Read the model definition and answer for the solid it produces. Units are mm, in the model's axes. Coordinates: 2 decimals unless noted, no trailing zeros.
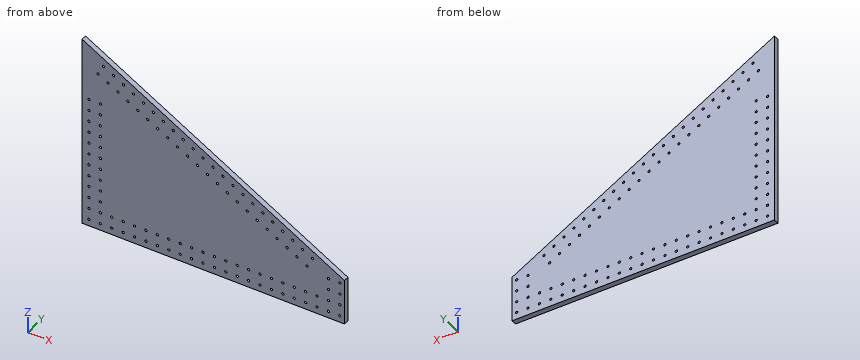
from build123d import *

# Parameters (mm, degrees)
F1_DEPTH = 12
F2_R     = 2.5527
F3_DEPTH = 508


with BuildPart() as f1:
    # F0 (on Front) → F1 (new body)
    with BuildSketch(Plane.XZ):
        Polygon((511.232538, -258.696949), (-72.967462, 69.018931), (-72.967462, -360.296949), (511.232538, -360.296949), align=None)
    extrude(amount=F1_DEPTH)

    # F2 (on face) → F3 (cut)
    with BuildSketch(Plane.XZ.offset(12)):
        with Locations((-57.714762, -345.044249)):
            Circle(F2_R)
        with Locations((-57.714762, -319.644249)):
            Circle(F2_R)
        with Locations((-57.714762, -294.244249)):
            Circle(F2_R)
        with Locations((-57.714762, -268.844249)):
            Circle(F2_R)
        with Locations((-57.714762, -243.444249)):
            Circle(F2_R)
        with Locations((-57.714762, -218.044249)):
            Circle(F2_R)
        with Locations((-57.714762, -192.644249)):
            Circle(F2_R)
        with Locations((-57.714762, -167.244249)):
            Circle(F2_R)
        with Locations((-57.714762, -141.844249)):
            Circle(F2_R)
        with Locations((-57.714762, -116.444249)):
            Circle(F2_R)
        with Locations((-57.714762, -91.044249)):
            Circle(F2_R)
        with Locations((-57.714762, -65.644249)):
            Circle(F2_R)
        with Locations((-32.314762, -345.044249)):
            Circle(F2_R)
        with Locations((-32.314762, -319.644249)):
            Circle(F2_R)
        with Locations((-32.314762, -294.244249)):
            Circle(F2_R)
        with Locations((-32.314762, -268.844249)):
            Circle(F2_R)
        with Locations((-32.314762, -243.444249)):
            Circle(F2_R)
        with Locations((-32.314762, -218.044249)):
            Circle(F2_R)
        with Locations((-32.314762, -192.644249)):
            Circle(F2_R)
        with Locations((-32.314762, -167.244249)):
            Circle(F2_R)
        with Locations((-32.314762, -141.844249)):
            Circle(F2_R)
        with Locations((-32.314762, -116.444249)):
            Circle(F2_R)
        with Locations((-32.314762, -91.044249)):
            Circle(F2_R)
        with Locations((-32.314762, -65.644249)):
            Circle(F2_R)
        with Locations((-6.914762, -319.644249)):
            Circle(F2_R)
        with Locations((-6.914762, -345.044249)):
            Circle(F2_R)
        with Locations((18.485238, -319.644249)):
            Circle(F2_R)
        with Locations((18.485238, -345.044249)):
            Circle(F2_R)
        with Locations((43.885238, -319.644249)):
            Circle(F2_R)
        with Locations((43.885238, -345.044249)):
            Circle(F2_R)
        with Locations((69.285238, -319.644249)):
            Circle(F2_R)
        with Locations((69.285238, -345.044249)):
            Circle(F2_R)
        with Locations((94.685238, -319.644249)):
            Circle(F2_R)
        with Locations((94.685238, -345.044249)):
            Circle(F2_R)
        with Locations((120.085238, -319.644249)):
            Circle(F2_R)
        with Locations((120.085238, -345.044249)):
            Circle(F2_R)
        with Locations((145.485238, -319.644249)):
            Circle(F2_R)
        with Locations((145.485238, -345.044249)):
            Circle(F2_R)
        with Locations((170.885238, -319.644249)):
            Circle(F2_R)
        with Locations((170.885238, -345.044249)):
            Circle(F2_R)
        with Locations((196.285238, -319.644249)):
            Circle(F2_R)
        with Locations((196.285238, -345.044249)):
            Circle(F2_R)
        with Locations((221.685238, -319.644249)):
            Circle(F2_R)
        with Locations((221.685238, -345.044249)):
            Circle(F2_R)
        with Locations((247.085238, -319.644249)):
            Circle(F2_R)
        with Locations((247.085238, -345.044249)):
            Circle(F2_R)
        with Locations((272.485238, -319.644249)):
            Circle(F2_R)
        with Locations((272.485238, -345.044249)):
            Circle(F2_R)
        with Locations((297.885238, -319.644249)):
            Circle(F2_R)
        with Locations((297.885238, -345.044249)):
            Circle(F2_R)
        with Locations((323.285238, -319.644249)):
            Circle(F2_R)
        with Locations((323.285238, -345.044249)):
            Circle(F2_R)
        with Locations((348.685238, -319.644249)):
            Circle(F2_R)
        with Locations((348.685238, -345.044249)):
            Circle(F2_R)
        with Locations((374.085238, -319.644249)):
            Circle(F2_R)
        with Locations((374.085238, -345.044249)):
            Circle(F2_R)
        with Locations((399.485238, -319.644249)):
            Circle(F2_R)
        with Locations((399.485238, -345.044249)):
            Circle(F2_R)
        with Locations((424.885238, -319.644249)):
            Circle(F2_R)
        with Locations((424.885238, -345.044249)):
            Circle(F2_R)
        with Locations((450.285238, -319.644249)):
            Circle(F2_R)
        with Locations((450.285238, -345.044249)):
            Circle(F2_R)
        with Locations((475.685238, -319.644249)):
            Circle(F2_R)
        with Locations((475.685238, -345.044249)):
            Circle(F2_R)
        with Locations((-25.048427, 24.649337)):
            Circle(F2_R)
        with Locations((-57.714762, 86.755751)):
            Circle(F2_R)
        with Locations((-32.314762, 86.755751)):
            Circle(F2_R)
        with Locations((501.085238, -319.644249)):
            Circle(F2_R)
        with Locations((501.085238, -345.044249)):
            Circle(F2_R)
        with Locations((-37.475226, 2.496806)):
            Circle(F2_R)
        with Locations((-2.895895, 12.222538)):
            Circle(F2_R)
        with Locations((-15.322695, -9.929994)):
            Circle(F2_R)
        with Locations((19.256636, -0.204262)):
            Circle(F2_R)
        with Locations((6.829836, -22.356794)):
            Circle(F2_R)
        with Locations((41.409168, -12.631062)):
            Circle(F2_R)
        with Locations((28.982368, -34.783593)):
            Circle(F2_R)
        with Locations((63.561699, -25.057861)):
            Circle(F2_R)
        with Locations((51.134899, -47.210393)):
            Circle(F2_R)
        with Locations((85.714231, -37.484661)):
            Circle(F2_R)
        with Locations((73.287431, -59.637192)):
            Circle(F2_R)
        with Locations((107.866762, -49.911461)):
            Circle(F2_R)
        with Locations((95.439962, -72.063992)):
            Circle(F2_R)
        with Locations((130.019294, -62.33826)):
            Circle(F2_R)
        with Locations((117.592494, -84.490792)):
            Circle(F2_R)
        with Locations((152.171825, -74.76506)):
            Circle(F2_R)
        with Locations((139.745025, -96.917591)):
            Circle(F2_R)
        with Locations((174.324356, -87.19186)):
            Circle(F2_R)
        with Locations((161.897557, -109.344391)):
            Circle(F2_R)
        with Locations((196.476888, -99.618659)):
            Circle(F2_R)
        with Locations((184.050088, -121.771191)):
            Circle(F2_R)
        with Locations((218.629419, -112.045459)):
            Circle(F2_R)
        with Locations((206.20262, -134.19799)):
            Circle(F2_R)
        with Locations((240.781951, -124.472258)):
            Circle(F2_R)
        with Locations((228.355151, -146.62479)):
            Circle(F2_R)
        with Locations((262.934482, -136.899058)):
            Circle(F2_R)
        with Locations((250.507683, -159.05159)):
            Circle(F2_R)
        with Locations((285.087014, -149.325858)):
            Circle(F2_R)
        with Locations((272.660214, -171.478389)):
            Circle(F2_R)
        with Locations((307.239545, -161.752657)):
            Circle(F2_R)
        with Locations((294.812746, -183.905189)):
            Circle(F2_R)
        with Locations((329.392077, -174.179457)):
            Circle(F2_R)
        with Locations((316.965277, -196.331988)):
            Circle(F2_R)
        with Locations((351.544608, -186.606257)):
            Circle(F2_R)
        with Locations((339.117809, -208.758788)):
            Circle(F2_R)
        with Locations((373.69714, -199.033056)):
            Circle(F2_R)
        with Locations((361.27034, -221.185588)):
            Circle(F2_R)
        with Locations((395.849671, -211.459856)):
            Circle(F2_R)
        with Locations((383.422872, -233.612387)):
            Circle(F2_R)
        with Locations((418.002203, -223.886656)):
            Circle(F2_R)
        with Locations((405.575403, -246.039187)):
            Circle(F2_R)
        with Locations((440.154734, -236.313455)):
            Circle(F2_R)
        with Locations((427.727935, -258.465987)):
            Circle(F2_R)
        with Locations((475.685238, -294.244249)):
            Circle(F2_R)
        with Locations((475.685238, -268.844249)):
            Circle(F2_R)
        with Locations((501.085238, -294.244249)):
            Circle(F2_R)
        with Locations((501.085238, -268.844249)):
            Circle(F2_R)
    extrude(amount=-F3_DEPTH, mode=Mode.SUBTRACT)


solid = f1.part
Q1. Straight lines are drawn through the part: probe 1 along X at (y, z) = (-9.75, -148); probe 2 along Z at (x, y) = (448, -4.5); probe 3 along X at (y, z) = (-7.5, -36). For each, find the intervals that lie inside material, in ascending order.
Findings below:
probe 1: x = -72.97 to 226.2, 230.51 to 282.91, 287.27 to 313.9
probe 2: z = -360.3 to -346.18, -343.91 to -320.78, -318.51 to -223.23
probe 3: x = -72.97 to 26.74, 31.23 to 83.64, 87.79 to 114.24
Q2. Flat-ended cylindrical pins translate along their axes: pin 1 Ø10 at (x, z) = (112, -88) entering from +Y; pin 2 Ø4 at (x, y) = (389, -7.5) entering from +Z. Find the tip coordinate at first contact, or state that the pin passes through.
Findings below:
pin 1: stops at y = 0
pin 2: stops at z = -189.01
Q3. A cutting plane is placed at A-A (y = -3.25). Count the separate pieces of the cut face and the enclosed holes in it, then the cut area to 3 significant figures.
Findings below:
separate pieces: 1
enclosed holes: 114
area: 153,000 mm2
